Part print with two shaded views. Sizes in mm from the minimum x, y, z corner. A direction names the side the tool comes from. Round coordinates to 2 decimals unless told otherwise and drop trailing zeros. Loops run counter-clockwise (first coordinate to the right, second up) from the corner with the lowest first, then second, coordinate; pieces in that order, holes last. Notation, with made-up numbers: (78, 75) -> (129, 75) arc R14 cw to (129, 92) -> close; hole circle Ø2 at (-23.5, 46). An arc over 180 degrees is marked (long way). Use a Markdown table: item, result. Add a question column.
Item 1: Which spindle directions (+Z, -Z, +X, -X, +Y, -Y) get a long thin tool onto all of the face, cutting with end or side? Do the marked faces 5, 6 and 7. Say none if no direction does.
Item 2: Probe line 1 (Y direction, x = 30, z = 17); line 2 (Y direction, x = 42, z = 27); line 3 (X direction, y = 1, z = 46.5). List the from-to ranges inside material, lowest first. Write a range as [from, to].
Item 3: Two-plate mould, pull along X, no slides. Class the marked faces 1, 2, 3 and 4: pulls with the +X half, pulls with the -X half, needs draft (parallel to the pull), parting line crosses it, or undercut.
Item 4: Flat gauge pins, fed straight in: pin 1 (10 mm diameter, centred on y = 19, z = 34, fed in from -X); pin 2 (1 mm diameter, centred on x = 30, z = 13, fed in from -Y); pin 3 (19.5 mm diameter, centred on x = 17.5, z = 7.5, fed in from -Y); pin 4 (10 mm diameter, centred on y = 4, z = 24.5, fed in from -X). Where does each tip first touch, or does it go through?
Item 5: Cut at A-A, the plane x = 17. List the corners of the cut face in (y, z).
Item 6: Cut at C-C, the plane y = 11.25. List the corners of the cut face in (x, z).
Item 7: Cut at D-D, the plane y = 17.25. List the corners of the cut face in (x, z), plus the area to 3 significant figures.
Item 8: Cut at B-B, the plane z = 40. List the corners of the cut face in (x, y).
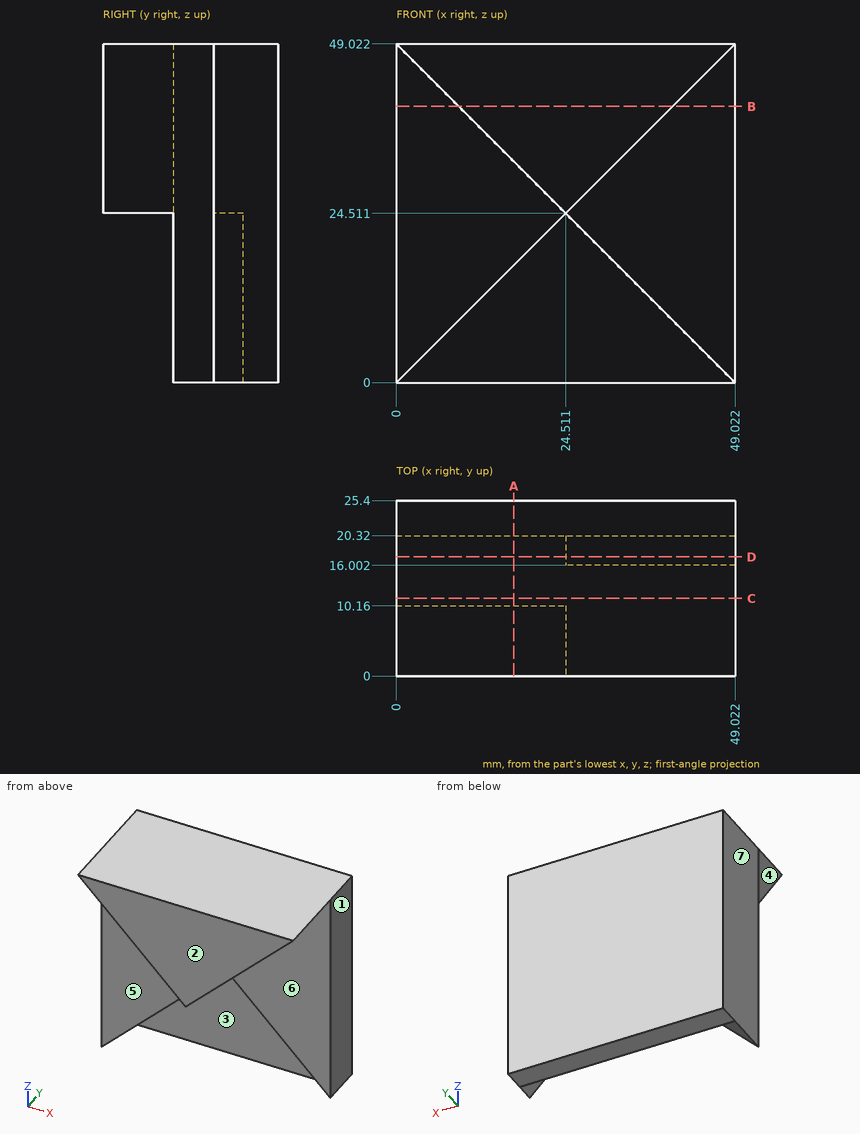
A:
| question | item | result |
|---|---|---|
| 1 | face 5 | -Z, -X, -Y |
| 1 | face 6 | -Z, +X, -Y |
| 1 | face 7 | +Z, -Z, -X, +Y, -Y |
| 2 | line 1 | y = [20.32, 25.4] |
| 2 | line 2 | y = [16, 25.4] |
| 2 | line 3 | x = [2.52, 46.5] |
| 3 | face 1 | pulls with the +X half |
| 3 | face 2 | needs draft |
| 3 | face 3 | undercut |
| 3 | face 4 | pulls with the -X half |
| 4 | pin 1 | stops at x = 0 |
| 4 | pin 2 | stops at y = 20.32 |
| 4 | pin 3 | stops at y = 10.16 |
| 4 | pin 4 | stops at x = 19.52 |
| 5 | outline | (0, 32.02) -> (10.16, 32.02) -> (10.16, 17) -> (20.32, 17) -> (20.32, 0) -> (25.4, 0) -> (25.4, 49.02) -> (0, 49.02) -> close |
| 6 | outline | (0, 0) -> (49.02, 49.02) -> (0, 49.02) -> close |
| 7 | outline | (0, 0) -> (24.51, 24.51) -> (49.02, 0) -> (49.02, 49.02) -> (0, 49.02) -> close |
| 7 | area | 1,800 mm^2 |
| 8 | outline | (0, 10.16) -> (9.02, 10.16) -> (9.02, 0) -> (40, 0) -> (40, 16) -> (49.02, 16) -> (49.02, 25.4) -> (0, 25.4) -> close |
